```python
from build123d import *

# Parameters (mm, degrees)
F1_DEPTH = 200
F3_D     = 10
F3_DEPTH = 50


with BuildPart() as f1:
    # F0 (on Front) → F1 (new body)
    with BuildSketch(Plane.XZ):
        Polygon((0, 50), (0, 0), (50, 0), (50, 50), (47, 50), (47, 3), (3, 3), (3, 50), align=None)
    extrude(amount=F1_DEPTH)

    # F3
    with Locations(Plane.YZ.offset(50)):
        with Locations((-180, 15), (-20, 15)):
            Hole(F3_D / 2, depth=F3_DEPTH)


solid = f1.part
```
CAD build for the part. Positions are in the model's coordinates, mm. A direction names the side the tool comes from. Round coordinates to 2 decimals unless told otherwise and drop trailing zeros. Order: outer loops, then holes, each group sorted by start corner. A loop starts at its lowest first (then second) coordinate and runs counter-clockwise, first axis right, second up.
Item 1: Probe line 1 along X through (y, z) = (-99, 33); line 2 along Z through (x, y) = (1, -20); line 3 along Z through (x, y) = (11.5, -16.5). List the from-to ranges inside material, lowest first.
Item 2: Saw through at D-D on y = -148.5. Write the cut outline in (x, z).
Item 3: Saw through at B-B on y = -180. Write the cut outline in (x, z).
Item 4: Tool access for faces 1 (the face through (3, -99, 26)), 2 (the face through (21, 0, 1)): list every direction of +Z, -Z, +X, -X, +Y, -Y with a clear straight run to the whole face (end or side of a thin tool).
Item 5: Pin check, flat tips, straight feed: pin 1 (6 mm diameter, centred on y = -180, z = 15, fed in from -X); pin 2 (2 mm diameter, centred on x = 31.5, y = -113, fed in from +Z). Stop position of each tip, or through.
Item 6: Mould opens along Z. For faces 3 (the face through (48, -176, 12)), 4 (the face through (0, -99, 25)), 5 (the face through (25, -99, 3)) say: pulls with the +Z half, pulls with the -Z half, needs draft (parallel to the pull), parting line crosses it, or undercut.
Item 7: Saw through at A-A on z = 43. Write the cut outline in (x, y).
Item 8: Saw through at C-C on z = 15. Write the cut outline in (x, y).
Reported:
1. line 1: x = 0 to 3, 47 to 50
1. line 2: z = 0 to 10, 20 to 50
1. line 3: z = 0 to 3
2. outline: (0, 0) - (50, 0) - (50, 50) - (47, 50) - (47, 3) - (3, 3) - (3, 50) - (0, 50) - close
3. outline: (0, 0) - (50, 0) - (50, 10) - (47, 10) - (47, 3) - (3, 3) - (3, 10) - (0, 10) - close; (0, 20) - (3, 20) - (3, 50) - (0, 50) - close; (47, 20) - (50, 20) - (50, 50) - (47, 50) - close
4. face 1: +Z, +Y, -Y
4. face 2: +Z, -Z, +X, -X, +Y
5. pin 1: passes through
5. pin 2: stops at z = 3
6. face 3: undercut
6. face 4: needs draft
6. face 5: pulls with the +Z half
7. outline: (0, -200) - (3, -200) - (3, 0) - (0, 0) - close; (47, -200) - (50, -200) - (50, 0) - (47, 0) - close
8. outline: (0, -200) - (3, -200) - (3, -185) - (0, -185) - close; (0, -175) - (3, -175) - (3, -25) - (0, -25) - close; (0, -15) - (3, -15) - (3, 0) - (0, 0) - close; (47, -200) - (50, -200) - (50, -185) - (47, -185) - close; (47, -175) - (50, -175) - (50, -25) - (47, -25) - close; (47, -15) - (50, -15) - (50, 0) - (47, 0) - close
